```python
from build123d import *

# Parameters (mm, degrees)
F0_R     = 35
F1_DEPTH = 5
F2_R     = 27
F2_R_2   = 25.5
F3_DEPTH = 5


with BuildPart() as f1:
    # F0 (on Top) → F1 (new body)
    with BuildSketch(Plane.XY):
        Circle(F0_R)
        with BuildLine():
            ThreePointArc((3, 32.3612422506), (22.9809703886, 22.9809703886), (32.3612422506, 3))
            ThreePointArc((32.3612422506, 3), (32.4652920297, 1.5016036189), (32.5, 0))
            ThreePointArc((32.5, 0), (32.4652920297, -1.5016036189), (32.3612422506, -3))
            ThreePointArc((32.3612422506, -3), (22.9809703886, -22.9809703886), (3, -32.3612422506))
            ThreePointArc((3, -32.3612422506), (0, -32.5), (-3, -32.3612422506))
            ThreePointArc((-3, -32.3612422506), (-22.9809703886, -22.9809703886), (-32.3612422506, -3))
            ThreePointArc((-32.3612422506, -3), (-32.5, 0), (-32.3612422506, 3))
            ThreePointArc((-32.3612422506, 3), (-22.9809703886, 22.9809703886), (-3, 32.3612422506))
            ThreePointArc((-3, 32.3612422506), (0, 32.5), (3, 32.3612422506))
        make_face(mode=Mode.SUBTRACT)
        with BuildLine():
            ThreePointArc((-6.7372564891, -3), (-7.2138024511, -1.5335185674), (-7.375, 0))
            ThreePointArc((-7.375, 0), (-7.2138024511, 1.5335185674), (-6.7372564891, 3))
            Line((-6.7372564891, 3), (-23.8117617996, 3))
            ThreePointArc((-23.8117617996, 3), (-24, 0), (-23.8117617996, -3))
            Line((-23.8117617996, -3), (-6.7372564891, -3))
        make_face()
        with BuildLine():
            ThreePointArc((-4.875, 0), (-3.4471455583, 3.4471455583), (0, 4.875))
            Line((0, 4.875), (0, 7.375))
            ThreePointArc((0, 7.375), (-1.5335185674, 7.2138024511), (-3, 6.7372564891))
            ThreePointArc((-3, 6.7372564891), (-5.2149125113, 5.2149125113), (-6.7372564891, 3))
            ThreePointArc((-6.7372564891, 3), (-7.2138024511, 1.5335185674), (-7.375, 0))
            Line((-7.375, 0), (-4.875, 0))
        make_face()
        with BuildLine():
            Line((0, -7.375), (0, -4.875))
            ThreePointArc((0, -4.875), (-3.4471455583, -3.4471455583), (-4.875, 0))
            Line((-4.875, 0), (-7.375, 0))
            ThreePointArc((-7.375, 0), (-7.2138024511, -1.5335185674), (-6.7372564891, -3))
            ThreePointArc((-6.7372564891, -3), (-5.2149125113, -5.2149125113), (-3, -6.7372564891))
            ThreePointArc((-3, -6.7372564891), (-1.5335185674, -7.2138024511), (0, -7.375))
        make_face()
        with BuildLine():
            Line((7.375, 0), (4.875, 0))
            ThreePointArc((4.875, 0), (3.4471455583, -3.4471455583), (0, -4.875))
            Line((0, -4.875), (0, -7.375))
            ThreePointArc((0, -7.375), (1.5335185674, -7.2138024511), (3, -6.7372564891))
            ThreePointArc((3, -6.7372564891), (5.2149125113, -5.2149125113), (6.7372564891, -3))
            ThreePointArc((6.7372564891, -3), (7.2138024511, -1.5335185674), (7.375, 0))
        make_face()
        with BuildLine():
            ThreePointArc((0, 4.875), (3.4471455583, 3.4471455583), (4.875, 0))
            Line((4.875, 0), (7.375, 0))
            ThreePointArc((7.375, 0), (7.2138024511, 1.5335185674), (6.7372564891, 3))
            ThreePointArc((6.7372564891, 3), (5.2149125113, 5.2149125113), (3, 6.7372564891))
            ThreePointArc((3, 6.7372564891), (1.5335185674, 7.2138024511), (0, 7.375))
            Line((0, 7.375), (0, 4.875))
        make_face()
        with BuildLine():
            ThreePointArc((-3, 6.7372564891), (-1.5335185674, 7.2138024511), (0, 7.375))
            ThreePointArc((0, 7.375), (1.5335185674, 7.2138024511), (3, 6.7372564891))
            Line((3, 6.7372564891), (3, 23.8117617996))
            ThreePointArc((3, 23.8117617996), (0, 24), (-3, 23.8117617996))
            Line((-3, 23.8117617996), (-3, 6.7372564891))
        make_face()
        with BuildLine():
            ThreePointArc((6.7372564891, 3), (7.2138024511, 1.5335185674), (7.375, 0))
            ThreePointArc((7.375, 0), (7.2138024511, -1.5335185674), (6.7372564891, -3))
            Line((6.7372564891, -3), (23.8117617996, -3))
            ThreePointArc((23.8117617996, -3), (23.9528942217, -1.502949901), (24, 0))
            ThreePointArc((24, 0), (23.9528942217, 1.502949901), (23.8117617996, 3))
            Line((23.8117617996, 3), (6.7372564891, 3))
        make_face()
        with BuildLine():
            ThreePointArc((3, -6.7372564891), (1.5335185674, -7.2138024511), (0, -7.375))
            ThreePointArc((0, -7.375), (-1.5335185674, -7.2138024511), (-3, -6.7372564891))
            Line((-3, -6.7372564891), (-3, -23.8117617996))
            ThreePointArc((-3, -23.8117617996), (0, -24), (3, -23.8117617996))
            Line((3, -23.8117617996), (3, -6.7372564891))
        make_face()
        with BuildLine():
            ThreePointArc((-3, 23.8117617996), (0, 24), (3, 23.8117617996))
            Line((3, 23.8117617996), (3, 25.3229145242))
            ThreePointArc((3, 25.3229145242), (0, 25.5), (-3, 25.3229145242))
            Line((-3, 25.3229145242), (-3, 23.8117617996))
        make_face()
        with BuildLine():
            ThreePointArc((-3, 25.3229145242), (0, 25.5), (3, 25.3229145242))
            Line((3, 25.3229145242), (3, 26.83281573))
            ThreePointArc((3, 26.83281573), (0, 27), (-3, 26.83281573))
            Line((-3, 26.83281573), (-3, 25.3229145242))
        make_face()
        with BuildLine():
            ThreePointArc((-3, 26.83281573), (0, 27), (3, 26.83281573))
            Line((3, 26.83281573), (3, 32.3612422506))
            ThreePointArc((3, 32.3612422506), (0, 32.5), (-3, 32.3612422506))
            Line((-3, 32.3612422506), (-3, 26.83281573))
        make_face()
        with BuildLine():
            Line((25.3229145242, 3), (23.8117617996, 3))
            ThreePointArc((23.8117617996, 3), (23.9528942217, 1.502949901), (24, 0))
            ThreePointArc((24, 0), (23.9528942217, -1.502949901), (23.8117617996, -3))
            Line((23.8117617996, -3), (25.3229145242, -3))
            ThreePointArc((25.3229145242, -3), (25.4556901337, -1.5026109997), (25.5, 0))
            ThreePointArc((25.5, 0), (25.4556901337, 1.5026109997), (25.3229145242, 3))
        make_face()
        with BuildLine():
            Line((26.83281573, 3), (25.3229145242, 3))
            ThreePointArc((25.3229145242, 3), (25.4556901337, 1.5026109997), (25.5, 0))
            ThreePointArc((25.5, 0), (25.4556901337, -1.5026109997), (25.3229145242, -3))
            Line((25.3229145242, -3), (26.83281573, -3))
            ThreePointArc((26.83281573, -3), (26.9581715321, -1.5023274094), (27, 0))
            ThreePointArc((27, 0), (26.9581715321, 1.5023274094), (26.83281573, 3))
        make_face()
        with BuildLine():
            Line((32.3612422506, 3), (26.83281573, 3))
            ThreePointArc((26.83281573, 3), (26.9581715321, 1.5023274094), (27, 0))
            ThreePointArc((27, 0), (26.9581715321, -1.5023274094), (26.83281573, -3))
            Line((26.83281573, -3), (32.3612422506, -3))
            ThreePointArc((32.3612422506, -3), (32.4652920297, -1.5016036189), (32.5, 0))
            ThreePointArc((32.5, 0), (32.4652920297, 1.5016036189), (32.3612422506, 3))
        make_face()
        with BuildLine():
            ThreePointArc((-23.8117617996, -3), (-24, 0), (-23.8117617996, 3))
            Line((-23.8117617996, 3), (-25.3229145242, 3))
            ThreePointArc((-25.3229145242, 3), (-25.5, 0), (-25.3229145242, -3))
            Line((-25.3229145242, -3), (-23.8117617996, -3))
        make_face()
        with BuildLine():
            ThreePointArc((-25.3229145242, -3), (-25.5, 0), (-25.3229145242, 3))
            Line((-25.3229145242, 3), (-26.83281573, 3))
            ThreePointArc((-26.83281573, 3), (-27, 0), (-26.83281573, -3))
            Line((-26.83281573, -3), (-25.3229145242, -3))
        make_face()
        with BuildLine():
            ThreePointArc((-26.83281573, -3), (-27, 0), (-26.83281573, 3))
            Line((-26.83281573, 3), (-32.3612422506, 3))
            ThreePointArc((-32.3612422506, 3), (-32.5, 0), (-32.3612422506, -3))
            Line((-32.3612422506, -3), (-26.83281573, -3))
        make_face()
        with BuildLine():
            ThreePointArc((3, -23.8117617996), (0, -24), (-3, -23.8117617996))
            Line((-3, -23.8117617996), (-3, -25.3229145242))
            ThreePointArc((-3, -25.3229145242), (0, -25.5), (3, -25.3229145242))
            Line((3, -25.3229145242), (3, -23.8117617996))
        make_face()
        with BuildLine():
            ThreePointArc((3, -25.3229145242), (0, -25.5), (-3, -25.3229145242))
            Line((-3, -25.3229145242), (-3, -26.83281573))
            ThreePointArc((-3, -26.83281573), (0, -27), (3, -26.83281573))
            Line((3, -26.83281573), (3, -25.3229145242))
        make_face()
        with BuildLine():
            ThreePointArc((3, -26.83281573), (0, -27), (-3, -26.83281573))
            Line((-3, -26.83281573), (-3, -32.3612422506))
            ThreePointArc((-3, -32.3612422506), (0, -32.5), (3, -32.3612422506))
            Line((3, -32.3612422506), (3, -26.83281573))
        make_face()
        with BuildLine():
            ThreePointArc((-25.3229145242, 3), (-18.0312229203, 18.0312229203), (-3, 25.3229145242))
            Line((-3, 25.3229145242), (-3, 26.83281573))
            ThreePointArc((-3, 26.83281573), (-19.091883092, 19.091883092), (-26.83281573, 3))
            Line((-26.83281573, 3), (-25.3229145242, 3))
        make_face()
        with BuildLine():
            ThreePointArc((3, 25.3229145242), (18.0312229203, 18.0312229203), (25.3229145242, 3))
            Line((25.3229145242, 3), (26.83281573, 3))
            ThreePointArc((26.83281573, 3), (19.091883092, 19.091883092), (3, 26.83281573))
            Line((3, 26.83281573), (3, 25.3229145242))
        make_face()
        with BuildLine():
            Line((26.83281573, -3), (25.3229145242, -3))
            ThreePointArc((25.3229145242, -3), (18.0312229203, -18.0312229203), (3, -25.3229145242))
            Line((3, -25.3229145242), (3, -26.83281573))
            ThreePointArc((3, -26.83281573), (19.091883092, -19.091883092), (26.83281573, -3))
        make_face()
        with BuildLine():
            Line((-3, -26.83281573), (-3, -25.3229145242))
            ThreePointArc((-3, -25.3229145242), (-18.0312229203, -18.0312229203), (-25.3229145242, -3))
            Line((-25.3229145242, -3), (-26.83281573, -3))
            ThreePointArc((-26.83281573, -3), (-19.091883092, -19.091883092), (-3, -26.83281573))
        make_face()
    extrude(amount=F1_DEPTH)

    # F2 (on face) → F3 (join)
    with BuildSketch(Plane.XY.offset(5)):
        Circle(F2_R)
        Circle(F2_R_2, mode=Mode.SUBTRACT)
    extrude(amount=F3_DEPTH)


solid = f1.part
```
For this review, take the finished solid that the model builds, in its own axes (mm). A direction names the side the tool comes from. Give positions to 0.01 mm unless a question says otherwise; leave off trailing zeros. Order: outer loops, then holes, each group sorted by start corner. A loop starts at its lowest first (then second) coordinate and runs counter-clockwise, first axis right, second up.
1) The part is to be moulded in two halves that separate along Y. For faces 3 (the face through (-16, 3, 2)), 4 (the face through (2, 29, 5)), say which applies: released by +Y, released by -Y, zero draft, split by the parting line, or undercut.
2) Wall thickness on line 1 (Y direction, x = 22.5, z = 2.5); line 2 (X direction, y = 7, z = 1); line 3 (Y direction, x = -28.5, z = 1.75): over which ranges is each line inside the solid? List them lowest first.
3) Take a section at C-C (z = 2). State how many separate pieces and enclosed holes the cut face has, then the cut area to 3 significant figures.
4) Take a section at B-B (x = -19). Give the boundary of the cut face in (y, z), then the cut area to 3 significant figures.
5) Take a section at D-D (z = 6). Give the boundary of the cut face in (x, y), then the cut area to 3 significant figures.
6) Take a section at A-A (y = -15.5). Give the boundary of the cut face in (x, z).
7) For faces 1 (the face through (24, -10, 10)), 2 (the face through (16, -3, 2)), list the 3-axis set-ups (+Z, -Z, +X, -X, +Y, -Y) from which the entire face can be reached by the end or side of a thin tool; tool diameter is ignored.
8) Insertion check: pin 1 (1 mm diameter, centred on x = -15, z = 7.5, fed in from -Y); pin 2 (1.5 mm diameter, centred on x = 28.5, z = 2, fed in from +Y); pin 3 (4 mm diameter, centred on x = 16, z = 2, fed in from -Y). Each pin has a flat end and moves straight along its axis. Give the tip position at first contact, or say it passes through.
Derived:
1. face 3: undercut
1. face 4: zero draft
2. line 1: y = -26.81 to -23.45, -14.92 to -12, -3 to 3, 12 to 14.92, 23.45 to 26.81
2. line 2: x = -34.29 to -31.74, -26.08 to -24.52, -3 to 3, 24.52 to 26.08, 31.74 to 34.29
2. line 3: y = -20.32 to -15.62, -3 to 3, 15.62 to 20.32
3. separate pieces: 1
3. enclosed holes: 9
3. area: 1,440 mm2
4. outline: (-29.39, 0) - (-26.37, 0) - (-26.37, 5) - (-29.39, 5) - close; (-19.18, 0) - (-17.01, 0) - (-17.01, 10) - (-19.18, 10) - close; (-3, 0) - (3, 0) - (3, 5) - (-3, 5) - close; (17.01, 0) - (19.18, 0) - (19.18, 10) - (17.01, 10) - close; (26.37, 0) - (29.39, 0) - (29.39, 5) - (26.37, 5) - close
4. area: 104 mm2
5. outline: circle Ø54 at (0, 0); hole circle Ø51 at (0, 0)
5. area: 247 mm2
6. outline: (-31.38, 0) - (-28.57, 0) - (-28.57, 5) - (-31.38, 5) - close; (-22.11, 0) - (-20.25, 0) - (-20.25, 10) - (-22.11, 10) - close; (-3, 0) - (3, 0) - (3, 5) - (-3, 5) - close; (20.25, 0) - (22.11, 0) - (22.11, 10) - (20.25, 10) - close; (28.57, 0) - (31.38, 0) - (31.38, 5) - (28.57, 5) - close
7. face 1: +Z, +X, -X, +Y, -Y
7. face 2: +Z, -Z
8. pin 1: stops at y = -22.78
8. pin 2: stops at y = 21.33
8. pin 3: stops at y = -32.08
